Check sheet for the modelled part. Datum: model origin and axes. Units: mm. A direction names the side the tool comes from. Round coordinates to 2 decimals unless told otherwise and drop trailing zeros. Write each loop counter-clockwise with the first axis right and the second up, starting at its lowest first coordinate (ties: lowest second). Pieces come first, ordered by that corner, then holes. Notation, with made-up numbers: (89.5, -14) -> (106.5, -14) arc R26 cw to (106.5, 1) -> close; hole circle Ø4 at (-17, 74). An arc over 180 degrees is marked (long way). One line per item, written item: value.
from build123d import *

# Parameters (mm, degrees)
EXTRUDE_THIN1_DEPTH     = 7
FILLET1_R               = 7
CUT_EXTRUDE1_DEPTH      = 10
CUT_EXTRUDE1_DEPTH_BACK = 10
SKETCH2_R               = 4
SKETCH3_R               = 2.25
BOSS_EXTRUDE1_DEPTH     = 1
FILLET2_R               = 5


with BuildPart() as part:
    # Sketch1 → Extrude-Thin1 (new, symmetric)
    with BuildSketch(Plane(origin=(0, 0, 0), x_dir=(0, 0, -1), z_dir=(1, 0, 0))):
        with BuildLine():
            Line((0, 0), (-15.070934652, 0))
            ThreePointArc((-15.070934652, 0), (-15.847391787, 0.102222521), (-16.570934652, 0.401923789))
            Line((-16.570934652, 0.401923789), (-20.374782229, 2.598076211))
            ThreePointArc((-20.374782229, 2.598076211), (-21.098325094, 2.897777479), (-21.874782229, 3))
            Line((-21.874782229, 3), (-35.874782229, 3))
            Line((-35.874782229, 3), (-35.874782229, 4))
            Line((-35.874782229, 4), (-21.874782229, 4))
            ThreePointArc((-21.874782229, 4), (-20.839506049, 3.863703305), (-19.874782229, 3.464101615))
            Line((-19.874782229, 3.464101615), (-16.070934652, 1.267949192))
            ThreePointArc((-16.070934652, 1.267949192), (-15.588572742, 1.068148347), (-15.070934652, 1))
            Line((-15.070934652, 1), (0, 1))
            Line((0, 1), (0, 0))
        make_face()
    extrude(amount=EXTRUDE_THIN1_DEPTH, both=True)

    # Fillet1
    fillet1_edges = [part.edges().sort_by_distance(p)[0] for p in [
        (-7, 3.5, 35.874782229),
        (7, 3.5, 35.874782229),
    ]]
    fillet(fillet1_edges, radius=FILLET1_R - 0.0001)  # a hair under: the kernel refuses the full size

    # Sketch2 → Cut-Extrude1 (cut, two sides: drawn at the far end of the back side and taken through both)
    with BuildSketch(Plane(origin=(0, 1, 0), x_dir=(1, 0, 0), z_dir=(0, 1, 0)).offset(-CUT_EXTRUDE1_DEPTH_BACK)):
        with Locations(Location((0, -28.874782229, 0), (0, 0, 90))):
            Circle(SKETCH2_R)
    extrude(amount=CUT_EXTRUDE1_DEPTH + CUT_EXTRUDE1_DEPTH_BACK, mode=Mode.SUBTRACT)

    # Sketch3 → Boss-Extrude1 (add)
    with BuildSketch(Plane.XZ):
        with BuildLine():
            Line((24, 0), (-24, 0))
            ThreePointArc((-24, 0), (-29, 5), (-24, 10))
            Line((-24, 10), (24, 10))
            ThreePointArc((24, 10), (29, 5), (24, 0))
        make_face()
        with Locations(Location((24, 5, 0), (0, 0, 270))):
            Circle(SKETCH3_R, mode=Mode.SUBTRACT)
        with Locations(Location((-24, 5, 0), (0, 0, 270))):
            Circle(SKETCH3_R, mode=Mode.SUBTRACT)
    extrude(amount=-BOSS_EXTRUDE1_DEPTH)

    # Fillet2
    fillet2_edges = [part.edges().sort_by_distance(p)[0] for p in [
        (-7, 0.5, 10),
        (7, 0.5, 10),
    ]]
    fillet(fillet2_edges, radius=FILLET2_R)


solid = part.part
Item 1: Sectioned sample at B-B (x = 20.5). Enter the section's corners in (y, z), then the cut area to 3 significant figures.
Result set:
outline: (0, 0) -> (1, 0) -> (1, 10) -> (0, 10) -> close
area: 10.0 mm^2
Item 2: Release check for a two-part mould opening along Z. For faces 6 (the cylindrical face through (21.804, 0.493, 5.488)), 7 (the flat face through (0, 0, 6)), 8 (the cylindrical face through (-26.196, 0.493, 5.488)), 9 (the cylindrical face through (-8.5, 0.49, 11.43)) record: pulls with the +Z half, pulls with the -Z half, needs draft (parallel to the pull), parting line crosses it, or undercut.
Result set:
face 6: undercut
face 7: needs draft
face 8: undercut
face 9: pulls with the +Z half
Item 3: Tool access check on faces 1 (the flat face through (-3, 4, 26)), 2 (the flat face through (7, 3.3, 21.9)), 3 (the flat face through (-7, 3.3, 21.9)), 4 (the flat face through (0, 1, 6)), 5 (the flat face through (-3, 3, 26)). Record the directions out of +Z, -Z, +X, -X, +Y, -Y that give a thin tool (end or side, any length) a straight path to the whole face; none if there is none.
Result set:
face 1: +Z, -Z, +X, -X, +Y
face 2: +Z, +X, +Y, -Y
face 3: +Z, -X, +Y, -Y
face 4: -Z, +X, -X, +Y
face 5: +Z, +X, -X, -Y
Item 4: Sectioned sample at A-A (z = 5). Enter the section's corners in (x, y).
Result set:
outline: (-29, 0) -> (-26.25, 0) -> (-26.25, 1) -> (-29, 1) -> close; (-21.75, 0) -> (21.75, 0) -> (21.75, 1) -> (-21.75, 1) -> close; (26.25, 0) -> (29, 0) -> (29, 1) -> (26.25, 1) -> close
Item 5: Depth check by flat-ended pin: pin 1 (1.5 mm diameter, centred on y = 0.5, z = 4, fed in from +X); pin 2 (2 mm diameter, centred on y = 1.5, z = 19.5, fed in from -X); pin 3 (0.8 mm diameter, centred on x = -19.5, y = 0.5, fed in from +Z); pin 4 (2 mm diameter, centred on y = 1.5, z = 22, fed in from +X). Enter the tip coordinate at first touch or a pass-through.
Result set:
pin 1: x = 28.99
pin 2: x = -7
pin 3: z = 10
pin 4: through
Item 6: Sectioned sample at C-C (z = 11.5). Enter the section's corners in (x, y), then the cut area to 3 significant figures.
Result set:
outline: (-8.43, 0) -> (8.43, 0) -> (8.43, 1) -> (-8.43, 1) -> close
area: 16.9 mm^2
Item 7: Material ranges on line 1 along X through (y, z) = (0.8, 5); line 2 along Z through (x, y) = (-0.5, 3.2); line 3 along Y through (x, z) = (4, 12), recorded low to high.
Result set:
line 1: -29 to -26.25, -21.75 to 21.75, 26.25 to 29
line 2: 19.42 to 24.91, 32.84 to 35.86
line 3: 0 to 1
